For this review, take the finished solid that the model builds, in its own axes (mm). Face numbers are marked on the shaded views. Round coordinates to 2 decimals unless told otherwise and drop trailing zeros. Order: outer loops, then holes, each group sorted by start corner. A loop starts at its lowest first (then second) coordinate and runs counter-clockwise, first axis right, second up. Notation, with made-up numbers: M -17.5,83.25 L 39.5,83.25 A14 ccw 39.5,92.25 Z; hole C 16.25,-5.5 d4. An arc over 180 degrees is marked long. Answer as a JSON object with one key per item and string values.
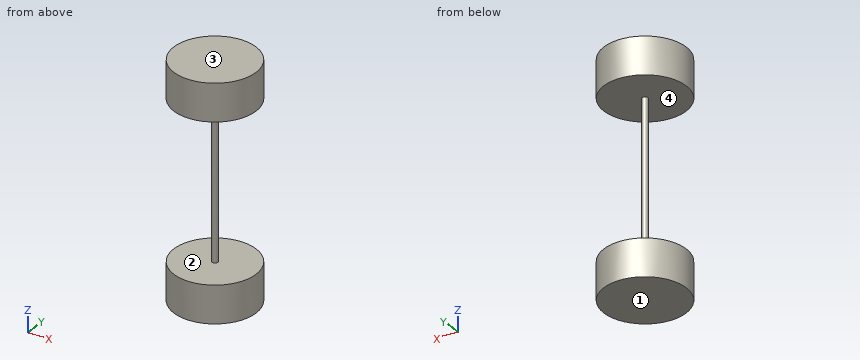
from build123d import *

# Parameters (mm, degrees)
F0_R     = 5.5
F1_DEPTH = 5
F3_R     = 5.5
F4_DEPTH = 5
F5_R     = 0.375
F6_DEPTH = 21


with BuildPart() as f1:
    # F0 (on Top) → F1 (new body)
    with BuildSketch(Plane.XY):
        Circle(F0_R)
    extrude(amount=F1_DEPTH)



with BuildPart() as f4:
    # F3 (on offset) → F4 (new body)
    with BuildSketch(Plane(origin=(0, 0, -21), x_dir=(1, 0, 0), z_dir=(0, 0, -1))):
        Circle(F3_R)
    extrude(amount=F4_DEPTH)


with BuildPart() as f1_1:
    add(f1.part)

    add(f4.part)  # F6 merges F4
    # F5 (on face) → F6 (join)
    with BuildSketch(Plane(origin=(0, 0, 0), x_dir=(1, 0, 0), z_dir=(0, 0, -1))):
        Circle(F5_R)
    extrude(amount=F6_DEPTH)


solid = f1_1.part
1) Add section B-B on x = 0. State the section outline as (y, z) points (3 decimals), and give its area (3 significant figures).
Geometry check:
{"outline": "M -5.5,-26 L 5.5,-26 L 5.5,-21 L 0.375,-21 L 0.375,0 L 5.5,0 L 5.5,5 L -5.5,5 L -5.5,0 L -0.375,0 L -0.375,-21 L -5.5,-21 Z", "area": "126 mm²"}
2) For L1, parallel to Z at x = -2.5, y = -2.5; L2, parallel to X at y = -0.25, z = 4.5; L3, parallel to Y at x = -4.75, z = -24, list the stretches that pass through material, from the lowest coordinate up.
Geometry check:
{"L1": "z = -26 to -21, 0 to 5", "L2": "x = -5.49 to 5.49", "L3": "y = -2.77 to 2.77"}
3) Add section D-D on x = -2.5. State the section outline as (y, z) points.
Geometry check:
{"outline": "M -4.9,-26 L 4.9,-26 L 4.9,-21 L -4.9,-21 Z; M -4.9,0 L 4.9,0 L 4.9,5 L -4.9,5 Z"}
4) Mouldability with a two-part tool opening along Z and no side actions: class the marked faces 1, 2, 3 and 4 as +Z half, -Z half, draft (parallel to the pull), parting line (faces both ways), or undercut.
Geometry check:
{"face 1": "-Z half", "face 2": "undercut", "face 3": "+Z half", "face 4": "undercut"}
5) Add section A-A on y = 2.75. State the section outline as (x, z) points.
Geometry check:
{"outline": "M -4.76,-26 L 4.76,-26 L 4.76,-21 L -4.76,-21 Z; M -4.76,0 L 4.76,0 L 4.76,5 L -4.76,5 Z"}
6) Insertion check: P1, Ø1, axis at x = -1, z = -22.5, coming from the -Y side. The pin has a flat end and moves straight along its axis. Give the tip position at first contact, or say it passes through.
Geometry check:
{"P1": "stops at y = -5.48"}
